The model under review builds one solid part; all positions refer to its coordinate system, in mm. Face numbers are marked on the shaded views. A direction names the side the tool comes from. Coordinates: 2 decimals unless noted, no trailing zeros. Order: outer loops, then holes, each group sorted by start corner. A loop starts at its lowest first (then second) coordinate and runs counter-clockwise, first axis right, second up. Notation, with made-up numbers: (24.25, 23) -> (71.25, 23) arc R28 cw to (71.25, 52) -> close; hole circle Ø4 at (36, 49). An arc over 180 degrees is marked (long way). Use one line per item in the form item = value.
from build123d import *

# Parameters (mm, degrees)
EXTRUDE_1_DEPTH     = 15.5
SKETCH_2_OUTSIDE_W  = 236.142
SKETCH_2_OUTSIDE_H  = 56.642
SKETCH_2_OUTSIDE_R  = 3
CUT_EXTRUDE_4_DEPTH = 10


with BuildPart() as part:
    # Эскиз1 → Вытянуть-Тонкостенный1 (new body)
    with BuildSketch(Plane.XY):
        Polygon((0, 0), (122.5, 0), (127.219413382, 4), (195, 4), (195, 2), (127.952959941, 2), (123.233546559, -2), (0, -2), align=None)
    extrude(amount=EXTRUDE_1_DEPTH)

    # Эскиз2 outside → Вырез-Вытянуть4 (cut)
    with BuildSketch(Plane(origin=(0, 4, 0), x_dir=(1, 0, 0), z_dir=(0, 1, 0))):
        with Locations((97.5, -7.75)):
            Rectangle(SKETCH_2_OUTSIDE_W, SKETCH_2_OUTSIDE_H)
        with BuildLine():
            Line((188.022623145, 0), (7.75, 0))
            ThreePointArc((7.75, 0), (0, -7.75), (7.75, -15.5))
            Line((7.75, -15.5), (188.022623145, -15.5))
            ThreePointArc((188.022623145, -15.5), (195.03841746, -7.75), (188.022623145, 0))
        make_face(mode=Mode.SUBTRACT)
        with Locations((187.25, -7.75)):
            Circle(SKETCH_2_OUTSIDE_R)
        with Locations((7.75, -7.75)):
            Circle(SKETCH_2_OUTSIDE_R)
    extrude(amount=-CUT_EXTRUDE_4_DEPTH, mode=Mode.SUBTRACT)


solid = part.part
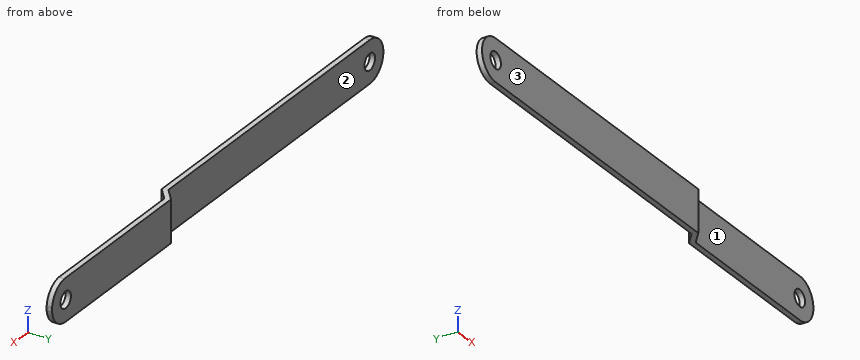
Item 1: To check wall thickness, follow L1, parallel to Z at x = 7.75, y = -1.4; L2, parallel to Y at x = 135, z = 10; L3, parallel to Y at x = 20, z = 11. State the ranges of each line that lie inside material, in increasing order. Write a range as from..to.
Results found:
L1 = 0..4.75, 10.75..15.5
L2 = 2..4
L3 = -2..0
Item 2: We need section A-A (z = 3). Write out the cut boundary in (x, y).
Results found:
outline = (1.63, -2) -> (123.23, -2) -> (127.95, 2) -> (193.42, 2) -> (193.42, 4) -> (127.22, 4) -> (122.5, 0) -> (1.63, 0) -> close
Item 3: Tool access review of the marked faces 1, 2 and 3: name each direction out of +Z, -Z, +X, -X, +Y, -Y from which nothing blocks a thin tool from reaching the whole face with its end or side.
Results found:
face_1 = +Z, -Z, +X, -Y
face_2 = +Z, -Z, -X, +Y
face_3 = +Z, -Z, +X, -X, -Y
Item 4: Clearance check with flat-ended pins moving along their axes: pin 1 (8 mm diameter, centred on x = 72, z = 11.5, fed in from +Y); pin 2 (8 mm diameter, centred on x = 177, z = 7, fed in from -Y); pin 3 (7 mm diameter, centred on x = 187.25, z = 7.75, fed in from +Y); pin 4 (1 mm diameter, centred on y = 3.5, z = 7.5, fed in from -X). State where each tip first meets the part, or that it passes through.
Results found:
pin_1 = 0
pin_2 = 2
pin_3 = 4
pin_4 = 126.04
Item 5: We need section B-B (x = 49.5). Write out the cut boundary in (y, z).
Results found:
outline = (-2, 0) -> (0, 0) -> (0, 15.5) -> (-2, 15.5) -> close
